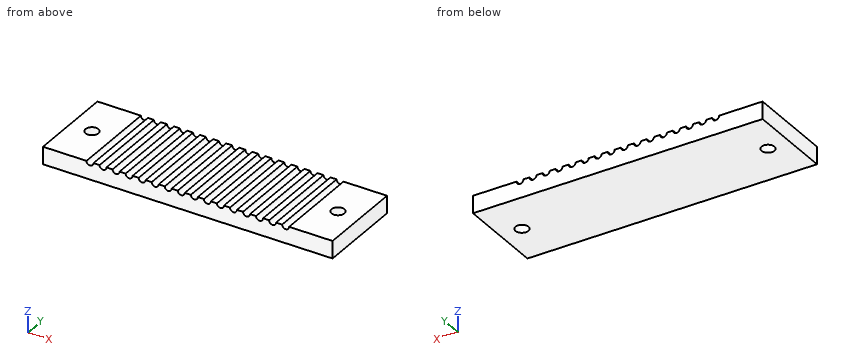
from build123d import *

# Parameters (mm, degrees)
EXTRUDE_1_DEPTH     = 20
SKETCH_2_R          = 1.5
CUT_EXTRUDE_1_DEPTH = 10


with BuildPart() as part:
    # 草图1 → 凸台-拉伸1 (new body)
    with BuildSketch(Plane(origin=(0, 0, 0), x_dir=(1, 0, 0), z_dir=(0, 1, 0))):
        with BuildLine():
            Line((-10.8, 0), (-0.8, 0))
            ThreePointArc((-0.8, 0), (0, 0.8), (0.8, 0))
            Line((0.8, 0), (2.2, 0))
            ThreePointArc((2.2, 0), (3, 0.8), (3.8, 0))
            Line((3.8, 0), (5.2, 0))
            ThreePointArc((5.2, 0), (6, 0.8), (6.8, 0))
            Line((6.8, 0), (8.2, 0))
            ThreePointArc((8.2, 0), (9, 0.8), (9.8, 0))
            Line((9.8, 0), (11.2, 0))
            ThreePointArc((11.2, 0), (12, 0.8), (12.8, 0))
            Line((12.8, 0), (14.2, 0))
            ThreePointArc((14.2, 0), (15, 0.8), (15.8, 0))
            Line((15.8, 0), (17.2, 0))
            ThreePointArc((17.2, 0), (18, 0.8), (18.8, 0))
            Line((18.8, 0), (20.2, 0))
            ThreePointArc((20.2, 0), (21, 0.8), (21.8, 0))
            Line((21.8, 0), (23.2, 0))
            ThreePointArc((23.2, 0), (24, 0.8), (24.8, 0))
            Line((24.8, 0), (26.2, 0))
            ThreePointArc((26.2, 0), (27, 0.8), (27.8, 0))
            Line((27.8, 0), (29.2, 0))
            ThreePointArc((29.2, 0), (30, 0.8), (30.8, 0))
            Line((30.8, 0), (32.2, 0))
            ThreePointArc((32.2, 0), (33, 0.8), (33.8, 0))
            Line((33.8, 0), (35.2, 0))
            ThreePointArc((35.2, 0), (36, 0.8), (36.8, 0))
            Line((36.8, 0), (38.2, 0))
            ThreePointArc((38.2, 0), (39, 0.8), (39.8, 0))
            Line((39.8, 0), (41.2, 0))
            ThreePointArc((41.2, 0), (42, 0.8), (42.8, 0))
            Line((42.8, 0), (44.2, 0))
            ThreePointArc((44.2, 0), (45, 0.8), (45.8, 0))
            Line((45.8, 0), (55.8, 0))
            Line((55.8, 0), (55.8, 4))
            Line((55.8, 4), (-10.8, 4))
            Line((-10.8, 4), (-10.8, 0))
        make_face()
    extrude(amount=EXTRUDE_1_DEPTH)

    # 草图2 → 切除-拉伸1 (cut)
    with BuildSketch(Plane.XY):
        with Locations((-5.8, 10)):
            Circle(SKETCH_2_R)
        with Locations((50.8, 10)):
            Circle(SKETCH_2_R)
    extrude(amount=-CUT_EXTRUDE_1_DEPTH, mode=Mode.SUBTRACT)


solid = part.part
Geometry check sheet. Reference: the model listing, model coordinates, mm. Round coordinates to 2 decimals unless told otherwise and drop trailing zeros. Order: outer loops, then holes, each group sorted by start corner. A loop starts at its lowest first (then second) coordinate and runs counter-clockwise, first axis right, second up. Notation, with made-up numbers: (6, 36.25) -> (12, 36.25) arc R24 cw to (12, 61.25) -> close; hole circle Ø5 at (-39.5, 26.5). An arc over 180 degrees is marked (long way). Use one line per item in the form item = value.
1. Cross-section at B-B, the plane x = 15. Enter the section's corners in (y, z).
Working result:
outline = (0, -4) -> (20, -4) -> (20, -0.8) -> (0, -0.8) -> close
2. Scan lines: line 1 along Y through (x, z) = (-5.8, -2.2); line 2 along X through (y, z) = (8.75, -3); line 3 along Y through (x, z) = (49.5, -0.5). Record each from-to range of solid material in increasing order. Write a range as from..to.
Working result:
line_1 = 0..8.5, 11.5..20
line_2 = -10.8..-6.63, -4.97..49.97, 51.63..55.8
line_3 = 0..9.25, 10.75..20
3. Go/stop test with a flat-tipped pin: pin 1 (2 mm diameter, centred on x = 9, z = -0.5, fed in from -Y). Record where the tip stops, or that it passes through.
Working result:
pin_1 = 0
4. Cross-section at A-A, the plane x = -5.8. Enter the section's corners in (y, z), plus the area to 3 significant figures.
Working result:
outline = (0, -4) -> (8.5, -4) -> (8.5, 0) -> (0, 0) -> close; (11.5, -4) -> (20, -4) -> (20, 0) -> (11.5, 0) -> close
area = 68.0 mm^2
